Geometry check sheet. Reference: the model listing, model coordinates, mm. Give positions to 0.01 mm unless a question says otherwise; leave off trailing zeros. Write each loop counter-clockwise with the first axis right and the second up, starting at its lowest first coordinate (ties: lowest second). Pieces come first, ordered by that corner, then holes. Notation, with made-up numbers: (45.25, 43) - (72.25, 43) arc R16 cw to (72.25, 56) - close; hole circle Ø4 at (50, 9). An arc over 180 degrees is marked (long way). Use a Markdown table: item, result.
```python
from build123d import *

# Parameters (mm, degrees)
SKETCH1_W           = 63.5
SKETCH1_H           = 82.55
SKETCH1_R           = 12.7
SKETCH1_R_2         = 2.0193
BOSS_EXTRUDE1_DEPTH = 3.175
SKETCH2_R           = 3.175
CUT_EXTRUDE1_DEPTH  = 4.175


with BuildPart() as part:
    # Sketch1 → Boss-Extrude1 (new body)
    with BuildSketch(Plane(origin=(0, 0, 0), x_dir=(1, 0, 0), z_dir=(0, 1, 0))):
        with Locations((31.75, 41.275)):
            Rectangle(SKETCH1_W, SKETCH1_H)
        with Locations((31.75, 50.8)):
            Circle(SKETCH1_R, mode=Mode.SUBTRACT)
        with Locations((9.752954744, 63.5)):
            Circle(SKETCH1_R_2, mode=Mode.SUBTRACT)
        with Locations((31.75, 76.2)):
            Circle(SKETCH1_R_2, mode=Mode.SUBTRACT)
        with Locations((53.747045256, 63.5)):
            Circle(SKETCH1_R_2, mode=Mode.SUBTRACT)
        with Locations((53.747045256, 38.1)):
            Circle(SKETCH1_R_2, mode=Mode.SUBTRACT)
        with Locations((31.75, 25.4)):
            Circle(SKETCH1_R_2, mode=Mode.SUBTRACT)
        with Locations((9.752954744, 38.1)):
            Circle(SKETCH1_R_2, mode=Mode.SUBTRACT)
    extrude(amount=BOSS_EXTRUDE1_DEPTH)

    # Sketch2 → Cut-Extrude1 (cut, through all)
    with BuildSketch(Plane(origin=(0, 3.175, 0), x_dir=(1, 0, 0), z_dir=(0, 1, 0))):
        with Locations((19.05, 12.7)):
            Circle(SKETCH2_R)
        with Locations((44.45, 12.7)):
            Circle(SKETCH2_R)
    extrude(amount=-CUT_EXTRUDE1_DEPTH, mode=Mode.SUBTRACT)


solid = part.part
```
1) Section check C-C on x = 31.75. Record the boundary of the cut face in (y, z) (3 decimals).
Working result:
| item | result |
|---|---|
| outline | (0, -82.55) - (3.175, -82.55) - (3.175, -78.219) - (0, -78.219) - close; (0, -74.181) - (3.175, -74.181) - (3.175, -63.5) - (0, -63.5) - close; (0, -38.1) - (3.175, -38.1) - (3.175, -27.419) - (0, -27.419) - close; (0, -23.381) - (3.175, -23.381) - (3.175, 0) - (0, 0) - close |
2) Section check B-B on z = -12.7. Record the boundary of the cut face in (x, y) (3 decimals), then the cut area to 3 significant figures.
Working result:
| item | result |
|---|---|
| outline | (0, 0) - (15.875, 0) - (15.875, 3.175) - (0, 3.175) - close; (22.225, 0) - (41.275, 0) - (41.275, 3.175) - (22.225, 3.175) - close; (47.625, 0) - (63.5, 0) - (63.5, 3.175) - (47.625, 3.175) - close |
| area | 161 mm² |
3) Section check D-D on y = 1.8. Count the separate pieces of the cut face and the enclosed holes in it, then the cut area to 3 significant figures.
Working result:
| item | result |
|---|---|
| separate pieces | 1 |
| enclosed holes | 9 |
| area | 4,600 mm² |
4) Mould release check, pull along Z, two halves, no side actions. Record for faces 1 (the flat face through (31, 2, 0)), 2 (the cylindrical face through (41.28, 1.61, -12.84)), 3 (the flat face through (31, 0, -33)): pulls with the +Z half, pulls with the -Z half, needs draft (parallel to the pull), parting line crosses it, or undercut.
Working result:
| item | result |
|---|---|
| face 1 | pulls with the +Z half |
| face 2 | undercut |
| face 3 | needs draft |
5) Section check A-A on z = -50.8. Record the boundary of the cut face in (x, y) (3 decimals), then the cut area to 3 significant figures.
Working result:
| item | result |
|---|---|
| outline | (0, 0) - (19.05, 0) - (19.05, 3.175) - (0, 3.175) - close; (44.45, 0) - (63.5, 0) - (63.5, 3.175) - (44.45, 3.175) - close |
| area | 121 mm² |
6) Material ranges on L1, parallel to Z at x = 31.75, y = 1; L2, parallel to X at y = 2.6, z = -12.5; L3, parallel to X at y = 2.65, z = -51.5, recorded low to high. Write a range as from..to.
Working result:
| item | result |
|---|---|
| L1 | z = -82.55..-78.22, -74.18..-63.5, -38.1..-27.42, -23.38..0 |
| L2 | x = 0..15.88, 22.22..41.28, 47.62..63.5 |
| L3 | x = 0..19.07, 44.43..63.5 |
